Autodesk Inventor part; units mm, degrees
ref_plane "YZ Plane" through (0, 0, 0) normal (1, 0, 0) x (0, 1, 0)
ref_plane "XZ Plane" through (0, 0, 0) normal (0, 1, 0) x (-1, 0, 0)
ref_plane "XY Plane" through (0, 0, 0) normal (0, 0, 1) x (1, 0, 0)
sketch "Sketch1" plane through (0, 0, 0) normal (0, 1, 0) x (-1, 0, 0)
  line L0 (-8, -4) -> (8, -4)
  line L1 (8, -4) -> (8, 4)
  line L2 (8, 4) -> (-8, 4)
  line L3 (-8, 4) -> (-8, -4)
  line L4 (-8, -4) -> (8, 4) construction
  line L5 (8, -4) -> (-8, 4) construction
  circle A0 centre (8, -4) radius 1
  circle A1 centre (8, -4) radius 2
  circle A2 centre (0, 4) radius 1
  circle A3 centre (-8, -4) radius 1
  circle A4 centre (-8, -4) radius 2
  circle A5 centre (0, 4) radius 2
  line L6 (8, -4) -> (0, 4)
  line L7 (0, 4) -> (-8, -4)
  line L8 (0, -4) -> (0, -5.5)
  line L9 (-6.6771, -5.5) -> (6.6771, -5.5)
  line L10 (4, 0) -> (5.0607, 1.0607)
  line L11 (-4, 0) -> (-5.0607, 1.0607)
  line L12 (0.1252, 5.9961) -> (9.9961, -3.8748)
  line L13 (-8.1282, -2.0445) -> (-1.9931, 4.1658)
  line L14 (-3.5251, -1.6464) -> (-0.3536, 1.5251)
  line L15 (3.5251, -1.6464) -> (0.3536, 1.5251)
  arc A6 (0.3536, 1.5251) -> (-0.3536, 1.5251) centre (0, 1.1716) ccw
  line L16 (3.1716, -2.5) -> (-3.1716, -2.5)
  arc A7 (-3.5251, -1.6464) -> (-3.1716, -2.5) centre (-3.1716, -2) ccw
  arc A8 (3.1716, -2.5) -> (3.5251, -1.6464) centre (3.1716, -2) ccw
  point P0 (0, 0)
  point P1 (0.1252, 5.9961)
  point P2 (-8.0861, -2.0019)
  point P3 (-6.6771, -5.5)
  point P4 (0.1252, 2.0039)
  point P5 (-0.1252, 2.0039)
  point P6 (1.9961, 4.1252)
  point P7 (8.1252, -2.0039)
  dimension "d0" = 16
  dimension "d1" = 8
  dimension "d2" = 2
  dimension "d3" = 4
  dimension "d4" = 2
  dimension "d5" = 2
  dimension "d6" = 4
  dimension "d7" = 4
  dimension "d8" = 1.5
  dimension "d9" = 1.5
  dimension "d10" = 1.5
  dimension "d23" = 90
  dimension "d28" = 90
  dimension "d29" = 0.5
  dimension "d31" = 0.5
  dimension "d32" = 1.5
  dimension "d33" = 1.5
  dimension "d34" = 1.5
  dimension "d35" = 90
extrude "Extrusion1" add sketch "Sketch1" along normal blind 1 contours A3 L7 A4 L0 | L0 A4 L3 A3 | L3 A4 L7 A3 | A4 L7 A5 L6 A1 L0 | L0 L8 L9 A4 | A4 L13 L3 | L3 L13 L11 L7 A4 | L0 A1 L9 L8 | L11 L13 L2 A5 L7 | A1 L6 A0 L0 | L0 A0 L1 A1 L12 | L7 A2 L6 A5 | A5 L2 A2 L7 | L6 L10 L12 L1 A1 | A1 L1 A0 L6 | L13 A5 L2 | A5 L12 L2 A2 | L6 A2 L2 A5 | A5 L2 L12 L10 L6 | L1 L12 A1 | A5 L12 L2 | A1 L12 | A5 L12
sketch "Sketch2" plane through (0, 1, 0) normal (0, 1, 0) x (1, 0, 0)
  line L0 (-8.1252, 2.0039) -> (-1.9961, -4.1252)
  arc A0 (-1.9961, -4.1252) -> (1.9931, -4.1658) centre (0, -4) ccw
  line L1 (1.9931, -4.1658) -> (8.0861, 2.0019)
  arc A1 (8.0861, 2.0019) -> (6.6771, 5.5) centre (8, 4) ccw
  line L2 (6.6771, 5.5) -> (-6.6771, 5.5)
  arc A2 (-6.6771, 5.5) -> (-8.1252, 2.0039) centre (-8, 4) ccw
  circle A3 centre (-8, 4) radius 1
  circle A4 centre (0, -4) radius 1
  circle A5 centre (8, 4) radius 1
  point P0 (0, 0)
extrude "Extrusion2" add sketch "Sketch2" along normal blind 1.5 and the other way blind 1 contours A3 | A5
sketch "Sketch4" plane through (0, 1, 0) normal (0, 1, 0) x (1, 0, 0)
  line L0 (-8.1252, 2.0039) -> (-1.9961, -4.1252)
  arc A0 (-1.9961, -4.1252) -> (1.9931, -4.1658) centre (0, -4) ccw
  line L1 (1.9931, -4.1658) -> (8.0861, 2.0019)
  arc A1 (8.0861, 2.0019) -> (6.6771, 5.5) centre (8, 4) ccw
  line L2 (6.6771, 5.5) -> (-6.6771, 5.5)
  arc A2 (-6.6771, 5.5) -> (-8.1252, 2.0039) centre (-8, 4) ccw
  circle A3 centre (-8, 4) radius 1
  circle A4 centre (8, 4) radius 1
  circle A5 centre (0, -4) radius 1
  line L3 (-3.1716, 2.5) -> (3.1716, 2.5)
  arc A6 (3.5251, 1.6464) -> (3.1716, 2.5) centre (3.1716, 2) ccw
  line L4 (3.5251, 1.6464) -> (0.3536, -1.5251)
  arc A7 (-0.3536, -1.5251) -> (0.3536, -1.5251) centre (0, -1.1716) ccw
  line L5 (-0.3536, -1.5251) -> (-3.5251, 1.6464)
  arc A8 (-3.1716, 2.5) -> (-3.5251, 1.6464) centre (-3.1716, 2) ccw
  point P0 (0, 0)
extrude "Extrusion4" add sketch "Sketch4" along normal blind 1.5 and the other way blind 1 contours A5
sketch "Sketch5" plane through (0, 1, 0) normal (0, 1, 0) x (1, 0, 0)
  line L0 (-8.1252, 2.0039) -> (-1.9961, -4.1252)
  arc A0 (-1.9961, -4.1252) -> (1.9931, -4.1658) centre (0, -4) ccw
  line L1 (1.9931, -4.1658) -> (8.0861, 2.0019)
  arc A1 (8.0861, 2.0019) -> (6.6771, 5.5) centre (8, 4) ccw
  line L2 (6.6771, 5.5) -> (-6.6771, 5.5)
  arc A2 (-6.6771, 5.5) -> (-8.1252, 2.0039) centre (-8, 4) ccw
  circle A3 centre (-8, 4) radius 1
  circle A4 centre (8, 4) radius 1
  circle A5 centre (0, -4) radius 1
  line L3 (-3.1716, 2.5) -> (3.1716, 2.5)
  arc A6 (3.5251, 1.6464) -> (3.1716, 2.5) centre (3.1716, 2) ccw
  line L4 (3.5251, 1.6464) -> (0.3536, -1.5251)
  arc A7 (-0.3536, -1.5251) -> (0.3536, -1.5251) centre (0, -1.1716) ccw
  line L5 (-0.3536, -1.5251) -> (-3.5251, 1.6464)
  arc A8 (-3.1716, 2.5) -> (-3.5251, 1.6464) centre (-3.1716, 2) ccw
  circle A9 centre (-4, 4) radius 1.5
  circle A10 centre (4, 4) radius 1.5
  point P0 (0, 0)
  dimension "d40" = 3
  dimension "d42" = 4
  dimension "d43" = 4
  dimension "d44" = 1.5
  dimension "d45" = 1.5
extrude "Extrusion5" add sketch "Sketch5" along normal blind 2 contours A10 | A9
sketch "Sketch6" plane through (-4, 3, -4) normal (0, 1, 0) x (1, 0, 0)
  circle A0 centre (0, 0) radius 1.5
  circle A1 centre (8, 0) radius 1.5
  circle A2 centre (0, 0) radius 1
  circle A3 centre (8, 0) radius 1
  point P0 (4, -4)
  dimension "d48" = 2
  dimension "d49" = 2
extrude "Extrusion6" add sketch "Sketch6" along normal blind 4 contours A2 | A3
equation "\"d2\" = d4"
equation "\"d3\" = d7"
equation "\"d5\" = d4"
equation "\"d6\" = d7"
equation "\"d45\" = d44"
equation "\"d49\" = d48"
properties part number "bar"
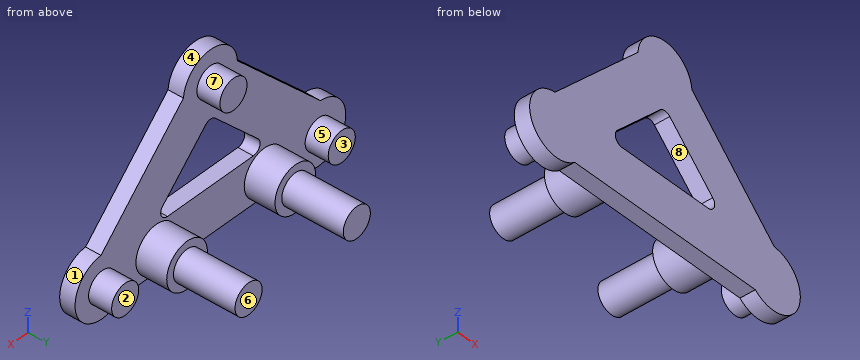
Could you check a few things on this model? Use its own coordinates, in mm. Face numbers are marked on the shaded views. A direction names the side the tool comes from. Coordinates: 2 decimals unless noted, no trailing zeros. Write each loop counter-clockwise with the first axis right and the second up, starting at its lowest first coordinate (ties: lowest second). Pieces come first, ordered by that corner, then holes. Notation, with made-up numbers: M 59,41 L 110,41 A18 ccw 110,48 Z; hole C 42.5,-22.75 d7. An arc over 180 degrees is marked long. Answer as CSV lines item,"result". Start each with the question number.
1) For the marked faces 1, 2, 3, 4 and 5, which set-ups out of +Z, -Z, +X, -X, +Y, -Y let a thin tool reach every point of the face, with its end or its side?
2) Please list where these lines run through material, in increasing order: line 1 (Y direction, x = 2.5, z = -2.75); line 2 (X direction, y = 6.25, z = -3.5); line 3 (Y direction, x = 8.5, z = -4.5). Write a range as from..to.
3) For P1, Ø0.5, axis at x = 1, y = 0.5, coming from the -Z side; P2, Ø2, axis at x = 8.5, z = -4, coming from the +Y side; P3, Ø0.5, axis at x = -1.5, y = 0.5, coming from the +Z side, each with a flat end and sliding along its axis, tell me the tip position at first contact or that it passes through.
4) I want a section at A-A, the plane y = 1.25. Please give me the cut outline in (x, z), and give its area (3 significant figures).
5) We'd pull the mould along Z, two halves only. Please class the marked faces 6, 7 and 8: +Z half, -Z half, draft (parallel to the pull), parting line (faces both ways), or undercut.
6) I want a section at C-C, the plane z = -4. Please give me the cut outline in (x, y), and give its area (3 significant figures).
7) I want a section at D-D, the plane z = -0.75. Please give me the cut outline in (x, y).
8) I want a section at B-B, the plane x = 0. Please give me the cut outline in (y, z), and give its area (3 significant figures).
Data:
1,face 1,"+Y, -Y"
1,face 2,"+Z, -Z, +X, +Y"
1,face 3,"+Z, -Z, -X, +Y"
1,face 4,"+Z, +Y, -Y"
1,face 5,"+Y"
2,line 1,"y = 0..1"
2,line 2,"x = -4.87..-3.13, 3.13..4.87"
2,line 3,"y = 0..2.5"
3,P1,"stops at z = -5.5"
3,P2,"stops at y = 2.5"
3,P3,"stops at z = 5.56"
4,outline,"C -8,-4 d2; C -4,-4 d3; C 0,4 d2; C 4,-4 d3; C 8,-4 d2"
4,area,"23.6 mm^2"
5,face 6,"draft"
5,face 7,"parting line"
5,face 8,"undercut"
6,outline,"M -10,0 L 10,0 L 10,1 L 9,1 L 9,2.5 L 7,2.5 L 7,1 L 5.5,1 L 5.5,3 L 5,3 L 5,7 L 3,7 L 3,3 L 2.5,3 L 2.5,1 L -2.5,1 L -2.5,3 L -3,3 L -3,7 L -5,7 L -5,3 L -5.5,3 L -5.5,1 L -7,1 L -7,2.5 L -9,2.5 L -9,1 L -10,1 Z"
6,area,"54.0 mm^2"
7,outline,"M -6.87,0 L -2.63,0 L -2.63,1 L -6.87,1 Z; M 2.63,0 L 6.85,0 L 6.85,1 L 2.63,1 Z"
8,outline,"M 0,-5.5 L 1,-5.5 L 1,-2.5 L 0,-2.5 Z; M 0,1.67 L 1,1.67 L 1,3 L 2.5,3 L 2.5,5 L 1,5 L 1,6 L 0,6 Z"
8,area,"10.3 mm^2"
